from build123d import *

# Parameters (mm, degrees)
F0_W     = 95.5
F0_H     = 95.5
F1_DEPTH = 0.2


with BuildPart() as f1:
    # F0 (on Top) → F1 (new body)
    with BuildSketch(Plane.XY):
        Polygon((1.5, -100), (100, -100), (100, -1.5), (100, 1.5), (100, 100), (1.5, 100), (-1.5, 100), (-100, 100), (-100, 1.5), (-100, -1.5), (-100, -100), (-1.5, -100), align=None)
        with Locations((-49.25, -49.25)):
            Rectangle(F0_W, F0_H, mode=Mode.SUBTRACT)
        with Locations((49.25, -49.25)):
            Rectangle(F0_W, F0_H, mode=Mode.SUBTRACT)
        with Locations((-49.25, 49.25)):
            Rectangle(F0_W, F0_H, mode=Mode.SUBTRACT)
        with Locations((49.25, 49.25)):
            Rectangle(F0_W, F0_H, mode=Mode.SUBTRACT)
    extrude(amount=F1_DEPTH)


solid = f1.part
Design review of the part built by this model. Coordinates are the model's own, in mm. Round coordinates to 2 decimals unless told otherwise and drop trailing zeros. Loops run counter-clockwise (first coordinate to the right, second up) from the corner with the lowest first, then second, coordinate; pieces in that order, holes last. Notation, with made-up numbers: (13.25, 15) -> (53.25, 15) arc R16 cw to (53.25, 21) -> close; hole circle Ø4 at (-24, -9). An arc over 180 degrees is marked (long way). Use one line per item in the form item = value. Start each with the question number.
Q1. Wall thickness on line 1 along X through (y, z) = (19, 0.1): over which ranges is the line inside the solid? List them lowest first. Write a range as [from, to].
Q2. We need section C-C on z = 0.1. Give the boundary of the cut face in (x, y).
Q3. We need section A-A on x = -57. Give the boundary of the cut face in (y, z).
Calculated:
q1.line_1 = [-100, -97], [-1.5, 1.5], [97, 100]
q2.outline = (-100, -100) -> (100, -100) -> (100, 100) -> (-100, 100) -> close; hole (-97, -97) -> (-1.5, -97) -> (-1.5, -1.5) -> (-97, -1.5) -> close; hole (-97, 1.5) -> (-1.5, 1.5) -> (-1.5, 97) -> (-97, 97) -> close; hole (1.5, -97) -> (97, -97) -> (97, -1.5) -> (1.5, -1.5) -> close; hole (1.5, 1.5) -> (97, 1.5) -> (97, 97) -> (1.5, 97) -> close
q3.outline = (-100, 0) -> (-97, 0) -> (-97, 0.2) -> (-100, 0.2) -> close; (-1.5, 0) -> (1.5, 0) -> (1.5, 0.2) -> (-1.5, 0.2) -> close; (97, 0) -> (100, 0) -> (100, 0.2) -> (97, 0.2) -> close
